Design review of the part built by this model. Coordinates are the model's own, in mm. A direction names the side the tool comes from. Round coordinates to 2 decimals unless told otherwise and drop trailing zeros. Loops run counter-clockwise (first coordinate to the right, second up) from the corner with the lowest first, then second, coordinate; pieces in that order, holes last. Notation, with made-up numbers: (27, 79.5) - (79, 79.5) arc R27 ccw to (79, 117.5) - close; hole circle Ø11 at (-1, -22). An arc over 180 degrees is marked (long way). Use one line per item in the form item = value. Start each with the question number.
(1) Wall thickness on probe 1 along X at (y, z) = (1.3, 0); probe 2 along Z at (x, y) = (0, 2.75); probe 3 along Z at (x, y) = (7, 2.85): over which ranges is each line inside the solid? List them lowest first. Write a range as [from, to].
(2) We need section D-D, the plane x = -7. Write out the cut boundary in (y, z), then the cut area to 3 significant figures.
(3) We need section B-B, the plane x = 0. Write out the cut boundary in (y, z).
(4) We need section C-C, the plane z = 0. Write out the cut boundary in (x, y), then the cut area to 3 significant figures.
(5) We need section A-A, the plane y = 0.45. Write out the cut boundary in (x, z), then the cut area to 3 significant figures.
(6) Machinability: for faces 5 (the cylindrical face through (0, 3, 1)), 6 (the flat face through (1, 2, 1)), which of the approach directions +Z, -Z, +X, -X, +Y, -Y give a long, thin tool a straight path to every point of the face, cutting with its end or side? Answer none if there is none.
(7) For pin 1 (4 mm diameter, centred on x = 0, z = 0, fed in from +Y); pin 2 (1.5 mm diameter, centred on x = 0.5, z = 0.5, fed in from -Y); pin 3 (2.5 mm diameter, centred on x = -7, z = 0, fed in from -Y), all flat-tipped, find the tip position at first contact; note any pin that passes through.
(8) The part is to be moulded in two halves that separate along X. For faces 1 (the flat face through (0, 2, 4)), 2 (the cylindrical face through (-8.5, 1.97, -0.07)), 3 (the cylindrical face through (-11.4, 1.97, 3.43)), 4 (the cylindrical face through (5.5, 1.97, -0.07)), say which applies: released by +X, released by -X, zero draft, split by the parting line, or undercut.
from build123d import *

# Parameters (mm, degrees)
BOSS_EXTRUDE1_DEPTH = 4
CUT_EXTRUDE1_REACH  = 6
SKETCH1_3_R         = 1
SKETCH1_3_R_2       = 1.5
SKETCH1_4_R         = 2.5
CUT_EXTRUDE2_DEPTH  = 2


with BuildPart() as part:
    # Sketch1 → Boss-Extrude1 (new body)
    with BuildSketch(Plane(origin=(0, 0, 0), x_dir=(1, 0, 0), z_dir=(0, 1, 0))):
        with BuildLine():
            Line((0, 4), (10, 4))
            ThreePointArc((10, 4), (11.414213562, 3.414213562), (12, 2))
            Line((12, 2), (12, -2))
            ThreePointArc((12, -2), (11.414213562, -3.414213562), (10, -4))
            Line((10, -4), (0, -4))
            Line((0, -4), (-10, -4))
            ThreePointArc((-10, -4), (-11.414213562, -3.414213562), (-12, -2))
            Line((-12, -2), (-12, 2))
            ThreePointArc((-12, 2), (-11.414213562, 3.414213562), (-10, 4))
            Line((-10, 4), (0, 4))
        make_face()
    extrude(amount=BOSS_EXTRUDE1_DEPTH)

    # Sketch1_3 → Cut-Extrude1 (cut, up to next)
    with BuildSketch(Plane(origin=(0, 0, 0), x_dir=(1, 0, 0), z_dir=(0, 1, 0)), mode=Mode.PRIVATE) as cut_extrude1_sk1:
        Circle(SKETCH1_3_R)
    cut_extrude1_tool1 = extrude(cut_extrude1_sk1.sketch, amount=CUT_EXTRUDE1_REACH, mode=Mode.PRIVATE) & part.part
    add(cut_extrude1_tool1.solids().sort_by_distance((0, 0, 0))[0], mode=Mode.SUBTRACT)
    # Sketch1_3 → Cut-Extrude1 (cut, up to next)
    with BuildSketch(Plane(origin=(0, 0, 0), x_dir=(1, 0, 0), z_dir=(0, 1, 0)), mode=Mode.PRIVATE) as cut_extrude1_sk2:
        with Locations((-7, 0)):
            Circle(SKETCH1_3_R_2)
    cut_extrude1_tool2 = extrude(cut_extrude1_sk2.sketch, amount=CUT_EXTRUDE1_REACH, mode=Mode.PRIVATE) & part.part
    add(cut_extrude1_tool2.solids().sort_by_distance((-7, 0, 0))[0], mode=Mode.SUBTRACT)
    # Sketch1_3 → Cut-Extrude1 (cut, up to next)
    with BuildSketch(Plane(origin=(0, 0, 0), x_dir=(1, 0, 0), z_dir=(0, 1, 0)), mode=Mode.PRIVATE) as cut_extrude1_sk3:
        with Locations((7, 0)):
            Circle(SKETCH1_3_R_2)
    cut_extrude1_tool3 = extrude(cut_extrude1_sk3.sketch, amount=CUT_EXTRUDE1_REACH, mode=Mode.PRIVATE) & part.part
    add(cut_extrude1_tool3.solids().sort_by_distance((7, 0, 0))[0], mode=Mode.SUBTRACT)

    # Sketch1_4 → Cut-Extrude2 (cut)
    with BuildSketch(Plane(origin=(0, 0, 0), x_dir=(1, 0, 0), z_dir=(0, 1, 0))):
        Circle(SKETCH1_4_R)
    extrude(amount=CUT_EXTRUDE2_DEPTH, mode=Mode.SUBTRACT)


solid = part.part
Data:
q1.probe_1 = [-12, -8.5], [-5.5, -2.5], [2.5, 5.5], [8.5, 12]
q1.probe_2 = [-4, -1], [1, 4]
q1.probe_3 = [-4, -1.5], [1.5, 4]
q2.outline = (0, -4) - (4, -4) - (4, -1.5) - (0, -1.5) - close; (0, 1.5) - (4, 1.5) - (4, 4) - (0, 4) - close
q2.area = 20.0 mm^2
q3.outline = (0, -4) - (4, -4) - (4, -1) - (2, -1) - (2, -2.5) - (0, -2.5) - close; (0, 2.5) - (2, 2.5) - (2, 1) - (4, 1) - (4, 4) - (0, 4) - close
q4.outline = (-12, 0) - (-8.5, 0) - (-8.5, 4) - (-12, 4) - close; (-5.5, 0) - (-2.5, 0) - (-2.5, 2) - (-1, 2) - (-1, 4) - (-5.5, 4) - close; (1, 2) - (2.5, 2) - (2.5, 0) - (5.5, 0) - (5.5, 4) - (1, 4) - close; (8.5, 0) - (12, 0) - (12, 4) - (8.5, 4) - close
q4.area = 58.0 mm^2
q5.outline = (-12, -2) arc R2 ccw to (-10, -4) - (10, -4) arc R2 ccw to (12, -2) - (12, 2) arc R2 ccw to (10, 4) - (-10, 4) arc R2 ccw to (-12, 2) - close; hole circle Ø3 at (-7, 0); hole circle Ø5 at (0, 0); hole circle Ø3 at (7, 0)
q5.area = 155 mm^2
q6.face_5 = +Y, -Y
q6.face_6 = -Y
q7.pin_1 = 4
q7.pin_2 = 2
q7.pin_3 = through
q8.face_1 = zero draft
q8.face_2 = undercut
q8.face_3 = released by -X
q8.face_4 = undercut
